Autodesk Inventor part; units mm, degrees
ref_plane "YZ Plane" through (0, 0, 0) normal (1, 0, 0) x (0, 1, 0)
ref_plane "XZ Plane" through (0, 0, 0) normal (0, 1, 0) x (-1, 0, 0)
ref_plane "XY Plane" through (0, 0, 0) normal (0, 0, 1) x (1, 0, 0)
sketch "Sketch1" plane through (0, 0, 0) normal (1, 0, 0) x (0, 1, 0)
  line L0 (0, 0) -> (10.3831, 0)
  line L1 (0, 0) -> (12.9478, 0)
  line L2 (0, 0) -> (100, 0)
  line L3 (100, 0) -> (100, -180)
  line L4 (80, -200) -> (20, -200)
  line L5 (0, -180) -> (0, 0)
  line L6 (20.0847, 0) -> (40.0847, 0)
  line L7 (60, 0) -> (80, 0)
  line L8 (80, 0) -> (80, -20)
  line L9 (70, -30) -> (70, -30)
  line L10 (60, -20) -> (60, 0)
  line L11 (40.0847, 0) -> (40.0847, -19)
  line L12 (30.0847, -29) -> (30.0847, -29)
  line L13 (0, 0) -> (0, -30)
  line L14 (20.0847, -19) -> (20.0847, 0)
  arc A0 (80, -200) -> (100, -180) centre (80, -180) ccw
  arc A1 (0, -180) -> (20, -200) centre (20, -180) ccw
  arc A2 (30.0847, -29) -> (40.0847, -19) centre (30.0847, -19) ccw
  arc A3 (20.0847, -19) -> (30.0847, -29) centre (30.0847, -19) ccw
  arc A4 (60, -20) -> (70, -30) centre (70, -20) ccw
  arc A5 (70, -30) -> (80, -20) centre (70, -20) ccw
  circle A6 centre (80, -180) radius 7.5
  circle A7 centre (20, -180) radius 7.5
  circle A8 centre (50, -120) radius 17.5
  circle A9 centre (50, -120) radius 32.5
  point P0 (100, -200)
  point P1 (0, -200)
  dimension "d0" = 100
  dimension "d1" = 200
  dimension "d10" = 20
  dimension "d16" = 20
  dimension "d23" = 15
  dimension "d24" = 35
  dimension "d25" = 65
  dimension "d26" = 50
  dimension "d31" = 80
extrude "Extrusion1" add sketch "Sketch1" along normal blind 20 contours L0 L1 L2 L14 A3 A2 L11 L10 A4 A5 L8 L3 A0 L4 A1 L5 | A9
extrude "Extrusion2" cut sketch "Sketch1" along normal blind 10 contours A8 | A9
properties part number "Wkp 01.03.1"
Here's how the part is built. I have some questions about the finished solid (model axes, mm). A direction names the side the tool comes from. Coordinates: 2 decimals unless noted, no trailing zeros. Write each loop counter-clockwise with the first axis right and the second up, starting at its lowest first coordinate (ties: lowest second). Pieces come first, ordered by that corner, then holes. Notation, with made-up numbers: (-2.75, -28) -> (28.25, -28) arc R24 cw to (28.25, 2) -> close; hole circle Ø8 at (46.5, -13.5). An arc over 180 degrees is marked (long way). Use a Markdown table: item, result. Add a question column.
(1) If we section it at A-A, the plane x = 13.5: Write out the boundary of the cut face in (y, z).
(2) If we section it at C-C, the plane y = 50: Write out the boundary of the cut face in (x, z), and give its area (3 significant figures).
(3) If we section it at B-B, the plane z = -120: Write out the boundary of the cut face in (x, y).
(4) I'm going to push a flat-ended pin straight in: P1, Ø4, axis at x = 16, y = 75, coming from the +Z side. Where does the tip first touch, or does it pass through?
(5) We'd pull the mould along Y, two halves only. Please class faces 4 (the flat face through (10, 100, -89)), 5 (the cylindrical face through (14.93, 47.72, -137.35)), 6 (the flat face through (10, 50, 0)): +Y half, -Y half, draft (parallel to the pull), parting line (faces both ways), or undercut.
(6) Please list where these lines run through material, in increasing order: line 1 (Y direction, x = 15.75, z = -17); line 2 (Z direction, x = 13, y = 50); line 3 (Y direction, x = 14.5, z = -120).
(7) For faces 1 (the cylindrical face through (4.93, 24.21, -100.22)), 2 (the flat face through (10, 0, -91)), 3 (the flat face through (10, 40.085, -9)), which set-ups out of +Z, -Z, +X, -X, +Y, -Y let a thin tool reach every point of the face, with its end or its side?
Outcome:
| question | item | result |
|---|---|---|
| 1 | outline | (0, -180) arc R20 ccw to (20, -200) -> (80, -200) arc R20 ccw to (100, -180) -> (100, 0) -> (80, 0) -> (80, -20) arc R10 cw to (60, -20) -> (60, 0) -> (40.08, 0) -> (40.08, -19) arc R10 cw to (20.08, -19) -> (20.08, 0) -> (0, 0) -> close; hole circle Ø15 at (20, -180); hole circle Ø35 at (50, -120); hole circle Ø15 at (80, -180) |
| 2 | outline | (0, -200) -> (20, -200) -> (20, -137.5) -> (10, -137.5) -> (10, -152.5) -> (0, -152.5) -> close; (0, -87.5) -> (10, -87.5) -> (10, -102.5) -> (20, -102.5) -> (20, 0) -> (0, 0) -> close |
| 2 | area | 3,000 mm^2 |
| 3 | outline | (0, 0) -> (20, 0) -> (20, 32.5) -> (10, 32.5) -> (10, 17.5) -> (0, 17.5) -> close; (0, 82.5) -> (10, 82.5) -> (10, 67.5) -> (20, 67.5) -> (20, 100) -> (0, 100) -> close |
| 4 | P1 | stops at z = -27.14 |
| 5 | face 4 | +Y half |
| 5 | face 5 | undercut |
| 5 | face 6 | draft |
| 6 | line 1 | y = 0 to 20.08, 40.08 to 60, 80 to 100 |
| 6 | line 2 | z = -200 to -137.5, -102.5 to 0 |
| 6 | line 3 | y = 0 to 32.5, 67.5 to 100 |
| 7 | face 1 | -X |
| 7 | face 2 | +Z, -Z, +X, -X, -Y |
| 7 | face 3 | +Z, +X, -X |
